CAD build for the part. Positions are in the model's coordinates, mm. A direction names the side the tool comes from. Give positions to 0.01 mm unless a question says otherwise; leave off trailing zeros. Order: outer loops, then holes, each group sorted by start corner. A loop starts at its lowest first (then second) coordinate and runs counter-clockwise, first axis right, second up. Notation, with made-up numbers: M -29.75,18.25 L 27.25,18.25 A18 ccw 27.25,44.25 Z; hole C 2.25,22 d2. An arc over 180 degrees is marked long. Put each result on its own line as item: value. Start each with the question number.
1) Cut at A-A (x = 42.5). Write the cut outline in (y, z).
2) Two-plate mould, pull along Y, no slides. Class faces 4 (the face through (0, 10, 0)), 5 (the face through (11.395, -0.381, 1.209)), 6 (the face through (12.498, -3.98, 12.637)): released by +Y, released by -Y, zero draft, split by the parting line, or undercut.
3) Drill centre lines: line 1 (Z direction, x = 21.5, y = -0.5); line 2 (Z direction, x = 53.5, y = 5.5); line 3 (Y direction, x = 13, z = -9.5). Where is each one in solid material? Low to high. Write a range as [from, to].
4) Tool access for faces 1 (the face through (76.2, 0, 0)), 2 (the face through (44.5, 7.7, -10.1)), 3 (the face through (3.72, 6.91, 3.91)): list every direction of +Z, -Z, +X, -X, +Y, -Y with a clear straight run to the whole face (end or side of a thin tool).
5) Pin check, flat tips, straight feed: pin 1 (2 mm diameter, centred on y = -2, z = 5.5, fed in from -X); pin 2 (6 mm diameter, centred on x = 49.5, z = -8, fed in from -Y); pin 3 (1.1 mm diameter, centred on y = 8, z = 0.5, fed in from -X); pin 4 (1 mm diameter, centred on y = 9, z = -3.5, fed in from -X). Stop position of each tip, or through.
```python
from build123d import *

# Parameters (mm, degrees)
HEX_2_DEPTH = 7.5438


with BuildPart() as part:
    # BodySke → BaseBody (revolve)
    with BuildSketch(Plane.XY, mode=Mode.PRIVATE) as basebody_sk:
        Polygon((0, 0), (0, 24.003), (0.127, 24.003), (13.129614107, 12.7), (74.93, 12.7), (76.2, 11.43), (76.2, 0), align=None)
    revolve(basebody_sk.sketch.rotate(Axis((0, 0, 0), (1, 0, 0)), 90), axis=Axis((0, 0, 0), (1, 0, 0)))  # turned: the seam where the file's is

    # Sketch2 → PreBroach (revolve, cut)
    with BuildSketch(Plane.XY, mode=Mode.PRIVATE) as prebroach_sk:
        Polygon((0, 7.9375), (7.5438, 7.9375), (12.126517762, 0), (0, 0), align=None)
    revolve(prebroach_sk.sketch.rotate(Axis((0, 0, 0), (1, 0, 0)), 90), axis=Axis((0, 0, 0), (1, 0, 0)), mode=Mode.SUBTRACT)  # turned: the seam where the file's is

    # Sketch3 → Hex 2 (cut)
    with BuildSketch(Plane.ZY):
        Polygon((-7.9375, -4.582717762), (-7.9375, 4.582717762), (0, 9.165435523), (7.9375, 4.582717762), (7.9375, -4.582717762), (0, -9.165435523), align=None)
    extrude(amount=-HEX_2_DEPTH, mode=Mode.SUBTRACT)


solid = part.part
```
Solution:
1. outline: C 0,0 d25.4
2. face 4: zero draft
2. face 5: undercut
2. face 6: split by the parting line
3. line 1: [-12.69, 12.69]
3. line 2: [-11.45, 11.45]
3. line 3: [-8.6, 8.6]
4. face 1: +Z, -Z, +X, +Y, -Y
4. face 2: +X
4. face 3: -X
5. pin 1: x = 8.17
5. pin 2: y = -11.67
5. pin 3: x = 7.54
5. pin 4: x = 0
